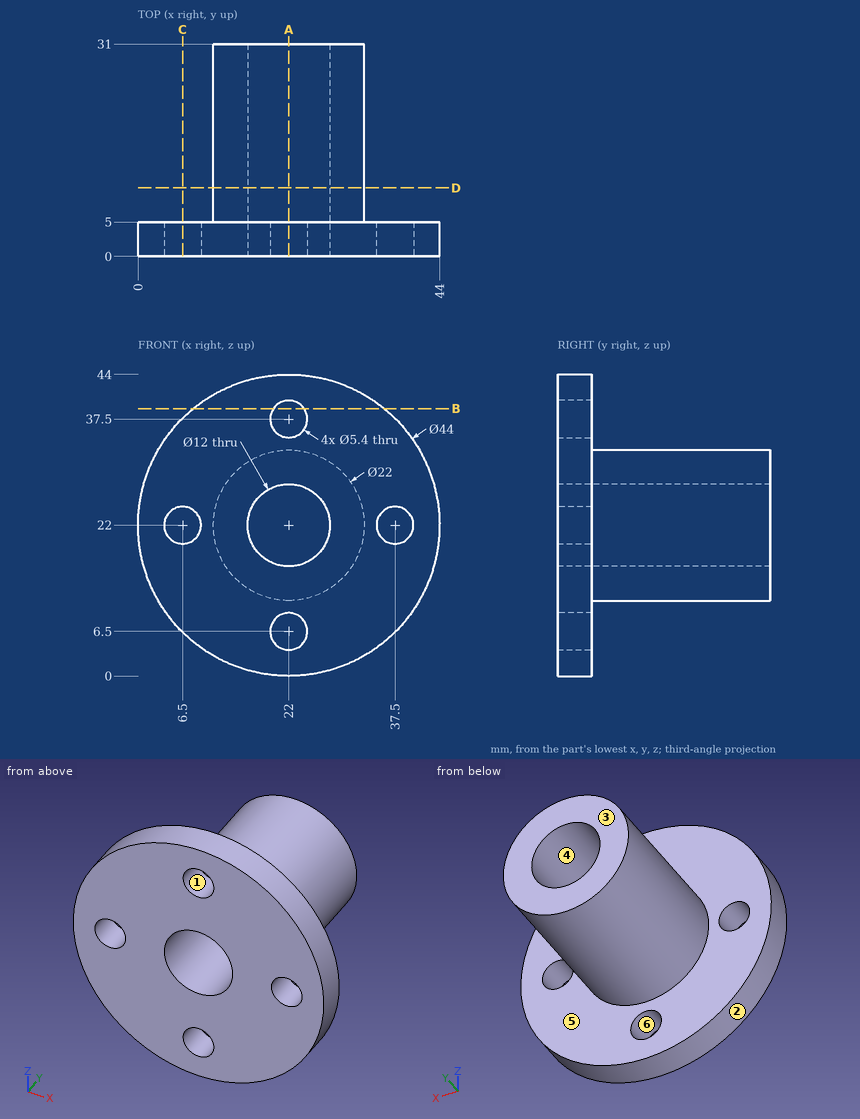
Part print with two shaded views. Sizes in mm from the minimum x, y, z corner. A direction names the side the tool comes from. Round coordinates to 2 decimals unless told otherwise and drop trailing zeros. Order: outer loops, then holes, each group sorted by start corner. A loop starts at its lowest first (then second) coordinate and runs counter-clockwise, first axis right, second up.
(1) Pin check, flat tips, straight feed: pin 1 (1.5 mm diameter, centred on y = 11, z = 26.5, fed in from +X); pin 2 (8.5 mm diameter, centred on x = 22, z = 37.5, fed in from +Y); pin 3 (12 mm diameter, centred on y = 3.5, z = 20, fed in from -X); pin 4 (8.5 mm diameter, centred on x = 22, z = 6.5, fed in from -Y). Stop position of each tip, or through.
(2) Band-saw the part on D-D (y = 10). List the corners of the cut face in (x, z), then the cut area to 3 significant figures.
(3) Band-saw the part on B-B (z = 39). List the corners of the cut face in (x, y) (3 decimals).
(4) Pull direction Z, two halves, no side cores. Call the marked faces 1, 2, 3 and 4: released by +Z, released by -Z, zero draft, split by the parting line, or undercut.
(5) Drill centre lines: line 1 (X direction, y = 3.6, z = 22); line 2 (Z direction, x = 22, y = 21); line 3 (Y direction, x = 32, z = 9). Where is each one in solid material? Low to high.
(6) Band-saw the part on C-C (x = 6.5). List the corners of the cut face in (y, z).
(7) 3-axis set-ups, long thin cutter, end or side, ignore diameter. For the marked faces 5 and 6: which of +Z, -Z, +X, -X, +Y, -Y reach the whole face in a straight line?
(8) Band-saw the part on A-A (x = 22). List the corners of the cut face in (y, z), then the cut area to 3 significant figures.
Verdict:
1. pin 1: stops at x = 32.34
1. pin 2: stops at y = 5
1. pin 3: stops at x = 0
1. pin 4: stops at y = 0
2. outline: circle Ø22 at (22, 22); hole circle Ø12 at (22, 22)
2. area: 267 mm2
3. outline: (8.036, 0) - (19.755, 0) - (19.755, 5) - (8.036, 5) - close; (24.245, 0) - (35.964, 0) - (35.964, 5) - (24.245, 5) - close
4. face 1: undercut
4. face 2: split by the parting line
4. face 3: zero draft
4. face 4: undercut
5. line 1: x = 0 to 3.8, 9.2 to 16, 28 to 34.8, 40.2 to 44
5. line 2: z = 11 to 16, 28 to 33
5. line 3: y = 0 to 5
6. outline: (0, 6.39) - (5, 6.39) - (5, 19.3) - (0, 19.3) - close; (0, 24.7) - (5, 24.7) - (5, 37.61) - (0, 37.61) - close
7. face 5: +Y
7. face 6: +Y, -Y
8. outline: (0, 0) - (5, 0) - (5, 3.8) - (0, 3.8) - close; (0, 9.2) - (5, 9.2) - (5, 11) - (31, 11) - (31, 16) - (0, 16) - close; (0, 28) - (31, 28) - (31, 33) - (5, 33) - (5, 34.8) - (0, 34.8) - close; (0, 40.2) - (5, 40.2) - (5, 44) - (0, 44) - close
8. area: 366 mm2
